from build123d import *

# Parameters (mm, degrees)
CROQUIS1_R              = 11
SALIENTE_EXTRUIR1_DEPTH = 15
CROQUIS3_R              = 5
SALIENTE_EXTRUIR2_DEPTH = 3
CROQUIS2_R              = 4.05
CORTAR_EXTRUIR1_DEPTH   = 289


with BuildPart() as part:
    # Croquis1 → Saliente-Extruir1 (new, symmetric)
    with BuildSketch(Plane.XY):
        Circle(CROQUIS1_R)
    extrude(amount=SALIENTE_EXTRUIR1_DEPTH, both=True)

    # Croquis3 → Saliente-Extruir2 (add)
    with BuildSketch(Plane.XY.offset(15)):
        Circle(CROQUIS3_R)
    extrude(amount=SALIENTE_EXTRUIR2_DEPTH)

    # Croquis2 → Cortar-Extruir1 (cut, symmetric)
    with BuildSketch(Plane.XY.offset(15)):
        Circle(CROQUIS2_R)
    extrude(amount=CORTAR_EXTRUIR1_DEPTH, both=True, mode=Mode.SUBTRACT)


solid = part.part
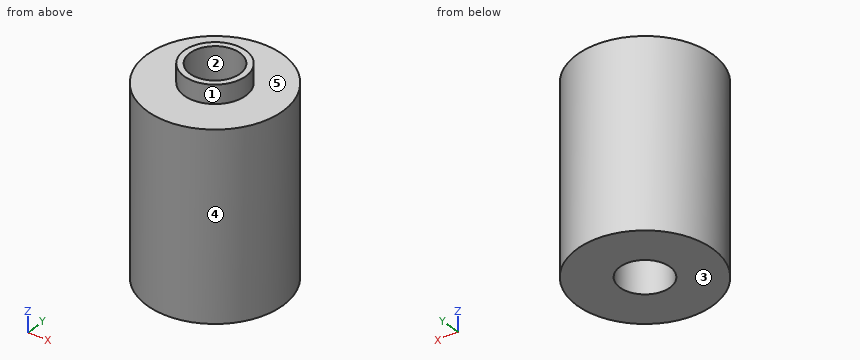
Design review of the part built by this model. Coordinates are the model's own, in mm. Face numbers are marked on the shaded views. A direction names the side the tool comes from. Coordinates: 2 decimals unless noted, no trailing zeros. Order: outer loops, then holes, each group sorted by start corner. A loop starts at its lowest first (then second) coordinate and runs counter-clockwise, first axis right, second up. Notation, with made-up numbers: M -31.5,49 L 24.5,49 A26 cw 24.5,67 Z; hole C 37.25,25.25 d6. An arc over 180 degrees is marked long. Use a Markdown table: item, result.
(1) For P1, Ø1, axis at y = -3.5, z = 13.5, coming from the -X side; P2, Ø4, axis at x = 2.5, z = 2, coming from the +Y side; P3, Ø4, axis at y = 2.5, z = 13.5, coming from the -X side; P4, Ø5, axis at x = -2.5, z = 5, coming from the -Y side, all flat-tipped, find the tip position at first contact; note any pin that passes through.
Worked answers:
| item | result |
|---|---|
| P1 | stops at x = -10.58 |
| P2 | stops at y = 10.99 |
| P3 | stops at x = -10.99 |
| P4 | stops at y = -11 |
(2) Draft analysis for pull direction X (two halves, no side actions). For the marked faces 1, 2 and 3, state which applies: released by +X, released by -X, zero draft, split by the parting line, or undercut.
Worked answers:
| item | result |
|---|---|
| face 1 | split by the parting line |
| face 2 | undercut |
| face 3 | zero draft |
(3) For the marked faces 4 and 5, list the 3-axis set-ups (+Z, -Z, +X, -X, +Y, -Y) from which the entire face can be reached by the end or side of a thin tool; tool diameter is ignored.
Worked answers:
| item | result |
|---|---|
| face 4 | +Z, -Z |
| face 5 | +Z |
(4) Add section A-A (x = 0). Give the boundary of the cut face in (y, z), then the cut area to 3 significant figures.
Worked answers:
| item | result |
|---|---|
| outline | M -11,-15 L -4.05,-15 L -4.05,18 L -5,18 L -5,15 L -11,15 Z; M 4.05,-15 L 11,-15 L 11,15 L 5,15 L 5,18 L 4.05,18 Z |
| area | 423 mm2 |
(5) Wall thickness on probe 1 along Y at (x, z) = (0, -2.5); probe 2 along Z at (x, y) = (1, 6.25); probe 3 along Y at (x, z) = (2.75, 8.5): over which ranges is each line inside the solid? List them lowest first.
Worked answers:
| item | result |
|---|---|
| probe 1 | y = -11 to -4.05, 4.05 to 11 |
| probe 2 | z = -15 to 15 |
| probe 3 | y = -10.65 to -2.97, 2.97 to 10.65 |
(6) Add section D-D (y = -8). Give the boundary of the cut face in (x, z), then the cut area to 3 significant figures.
Worked answers:
| item | result |
|---|---|
| outline | M -7.55,-15 L 7.55,-15 L 7.55,15 L -7.55,15 Z |
| area | 453 mm2 |
(7) Add section C-C (z = 3.5). Give the boundary of the cut face in (x, y).
Worked answers:
| item | result |
|---|---|
| outline | C 0,0 d22; hole C 0,0 d8.1 |
